```python
from build123d import *

# Parameters (mm, degrees)
F1_DEPTH = 5


with BuildPart() as f1:
    # F0 (on Front) → F1 (new body)
    with BuildSketch(Plane.XZ):
        Polygon((-60.1411065459, 94.3177779019), (-60.1411065459, -25.6822220981), (59.8588934541, -25.6822220981), (59.8588934541, -10.6822220981), (59.8588934541, 4.3177779019), (59.8588934541, 94.3177779019), (34.8588934541, 94.3177779019), (34.8588934541, 4.3177779019), (-35.1411065459, 4.3177779019), (-35.1411065459, 94.3177779019), align=None)
        with BuildLine():
            ThreePointArc((-32.1499717459, -10.6822220981), (-30.1411065459, -8.6733568981), (-28.132241346, -10.6822220981))
            ThreePointArc((-28.132241346, -10.6822220981), (-30.1411065459, -12.6910872981), (-32.1499717459, -10.6822220981))
        make_face(mode=Mode.SUBTRACT)
        with BuildLine():
            ThreePointArc((27.8374452822, -10.6822220981), (29.8588934541, -8.6607739263), (31.8803416259, -10.6822220981))
            ThreePointArc((31.8803416259, -10.6822220981), (29.8588934541, -12.70367027), (27.8374452822, -10.6822220981))
        make_face(mode=Mode.SUBTRACT)
    extrude(amount=F1_DEPTH)


solid = f1.part
```
The listing builds one solid part. Answer for the finished solid, in the listing's coordinates (mm). A direction names the side the tool comes from. Coordinates: 2 decimals unless noted, no trailing zeros. Loops run counter-clockwise (first coordinate to the right, second up) from the corner with the lowest first, then second, coordinate; pieces in that order, holes last. Notation, with made-up numbers: (41.25, 65) -> (100.25, 65) arc R11 cw to (100.25, 78) -> close; hole circle Ø5 at (56, 51.25). An arc over 180 degrees is marked (long way). Use one line per item in the form item = value. Start each with the question number.
Item 1: The mould has two halves that part along X. Classify faces 1 (the face through (-60.141, -2, 35)), 2 (the face through (48, -2, 94.318)), 3 (the face through (34.859, -2, 50)): released by +X, released by -X, zero draft, split by the parting line, or undercut.
Item 2: The part is cut by section A-A on y = -0.85. Determine the outline of the cut face in (x, z), then the cut area to 3 significant figures.
Item 3: Consider L1, parallel to X at y = -1.4, z = 80; L2, parallel to Z at x = -30.5, y = -4.4; L3, parallel to X at y = -2.35, z = -10.5. Determine where each line is inside the solid, lowest interval first. Write a range as [from, to].
Item 4: The part is cut by section B-B on z = 27. Determine the outline of the cut face in (x, y).
Item 5: A tool of negligible diameter and unlimited length cuts with its end or side. For faces 4 (the face through (-35.141, -2, 49)), 5 (the face through (-1, -5, -5)), from which of +Z, -Z, +X, -X, +Y, -Y can it reach the whole face along a straight path? Write none if from no direction.
Item 6: The part is cut by section C-C on x = -3. Determine the outline of the cut face in (y, z).
Answer key:
q1.face_1 = released by -X
q1.face_2 = zero draft
q1.face_3 = undercut
q2.outline = (-60.14, -25.68) -> (59.86, -25.68) -> (59.86, 94.32) -> (34.86, 94.32) -> (34.86, 4.32) -> (-35.14, 4.32) -> (-35.14, 94.32) -> (-60.14, 94.32) -> close; hole circle Ø4.02 at (-30.14, -10.68); hole circle Ø4.04 at (29.86, -10.68)
q2.area = 8,070 mm2
q3.L1 = [-60.14, -35.14], [34.86, 59.86]
q3.L2 = [-25.68, -12.66], [-8.71, 4.32]
q3.L3 = [-60.14, -32.14], [-28.14, 27.85], [31.87, 59.86]
q4.outline = (-60.14, -5) -> (-35.14, -5) -> (-35.14, 0) -> (-60.14, 0) -> close; (34.86, -5) -> (59.86, -5) -> (59.86, 0) -> (34.86, 0) -> close
q5.face_4 = +Z, +Y, -Y
q5.face_5 = +Z, -Z, +X, -X, -Y
q6.outline = (-5, -25.68) -> (0, -25.68) -> (0, 4.32) -> (-5, 4.32) -> close
